CAD build for the part. Positions are in the model's coordinates, mm. Face numbers are marked on the shaded views. A direction names the side the tool comes from. Coordinates: 2 decimals unless noted, no trailing zeros. Write each loop counter-clockwise with the first axis right and the second up, starting at its lowest first coordinate (ties: lowest second). Pieces come first, ordered by that corner, then holes. Notation, with made-up numbers: M 0,31 L 38,31 A13 ccw 38,43 Z; hole C 18,60.25 d7. An arc over 180 degrees is marked long. Put each result on its own line as item: value. Start each with the question number.
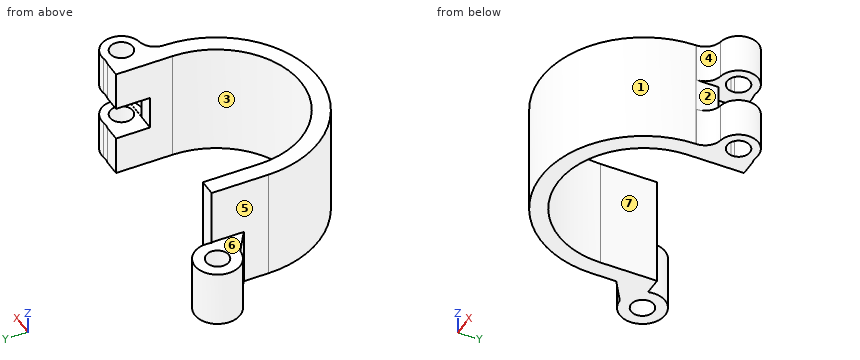
```python
from build123d import *

# Parameters (mm, degrees)
SKETCH1_R                           = 4
SKETCH1_R_2                         = 2
BOSS_EXTRUDE1_DEPTH                 = 10
BOSS_EXTRUDE2_DEPTH                 = 20
BOSS_EXTRUDE3_DEPTH                 = 10
SKETCH5_R                           = 3.5
SKETCH5_R_2                         = 2
BOSS_EXTRUDE4_DEPTH                 = 20
SKETCH4_W                           = 6
SKETCH4_H                           = 6.000142194
CUT_EXTRUDE1_DEPTH                  = 3
CUT_EXTRUDE1_DIRECTION_2_REACH      = 323.185
CUT_EXTRUDE1_DIRECTION_2_END_RADIUS = 3.5
FILLET2_R                           = 3
SKETCH6_W                           = 4.423537042
SKETCH6_H                           = 5.967206981
CUT_EXTRUDE2_DEPTH                  = 36.49639057
BODY_MOVE_COPY1_OUTLINE_R           = 2
BODY_MOVE_COPY1_DEPTH               = 10
BODY_MOVE_COPY1_START               = 2.967206981
BODY_MOVE_COPY1_2_DEPTH             = 0.032793019
BODY_MOVE_COPY1_START_2             = -10
BODY_MOVE_COPY1_3_OUTLINE_R         = 2
BODY_MOVE_COPY1_3_DEPTH             = 10
BODY_MOVE_COPY1_START_3             = -3
BODY_MOVE_COPY1_4_DEPTH             = 0.032793019


# Read off the part's stored shape, not the designer's step: Body-Move/Copy1
with BuildPart() as part:
    # Sketch1 → Boss-Extrude1 (new body)
    with BuildSketch(Plane.XY):
        with Locations(Location((-22, -289, 0), (0, 0, 270))):
            Circle(SKETCH1_R)
        with Locations(Location((-22, -289, 0), (0, 0, 270))):
            Circle(SKETCH1_R_2, mode=Mode.SUBTRACT)
    extrude(amount=BOSS_EXTRUDE1_DEPTH)



with BuildPart() as body_2:
    # Sketch2 → Boss-Extrude2 (new body)
    with BuildSketch(Plane.XY.offset(10)):
        with BuildLine():
            Line((-18, -300), (-18, -295.71047836))
            Line((-18, -295.71047836), (-18, -290))
            Line((-18, -290), (-15, -290))
            Line((-15, -290), (-15, -300))
            ThreePointArc((-15, -300), (0, -315), (15, -300))
            Line((15, -300), (15, -290))
            Line((15, -290), (18, -290))
            Line((18, -290), (18, -300))
            ThreePointArc((18, -300), (0, -318), (-18, -300))
        make_face()
    extrude(amount=-BOSS_EXTRUDE2_DEPTH)


with BuildPart() as part_1:
    add(part.part)

    add(body_2.part)  # Boss-Extrude3 merges body 2
    # Sketch3 → Boss-Extrude3 (add)
    with BuildSketch(Plane.XY.offset(10)):
        Polygon((-18, -290), (-18.290403154, -290), (-22, -293), (-18, -295.669919522), align=None)
    extrude(amount=-BOSS_EXTRUDE3_DEPTH)

    # Sketch5 → Boss-Extrude4 (add)
    with BuildSketch(Plane.XY.offset(10)):
        with Locations((19.974192434, -293.5)):
            Circle(SKETCH5_R)
        with Locations((19.974192434, -293.5)):
            Circle(SKETCH5_R_2, mode=Mode.SUBTRACT)
    extrude(amount=-BOSS_EXTRUDE4_DEPTH)

    # Sketch4 → Cut-Extrude1 (cut)
    with BuildSketch(Plane(origin=(18, 0, 0), x_dir=(0, 0, -1), z_dir=(1, 0, 0))):
        with Locations((0, -293.000071097)):
            Rectangle(SKETCH4_W, SKETCH4_H)
    extrude(amount=-CUT_EXTRUDE1_DEPTH, mode=Mode.SUBTRACT)

    # Cut-Extrude1 direction 2: up to this cylinder (the profile starts inside it)
    cut_extrude1_direction_2_end = Plane(origin=(19.974192434, -293.5, 0), z_dir=(0, 0, 1)) * Cylinder(CUT_EXTRUDE1_DIRECTION_2_END_RADIUS, 654.37, mode=Mode.PRIVATE)
    # Sketch4 → Cut-Extrude1 direction 2 (cut, up to the surface)
    with BuildSketch(Plane(origin=(18, 0, 0), x_dir=(0, 0, -1), z_dir=(1, 0, 0)), mode=Mode.PRIVATE) as cut_extrude1_direction_2_sk1:
        with Locations((0, -293.000071097)):
            Rectangle(SKETCH4_W, SKETCH4_H)
    cut_extrude1_direction_2_tool1 = extrude(cut_extrude1_direction_2_sk1.sketch, amount=CUT_EXTRUDE1_DIRECTION_2_REACH, mode=Mode.PRIVATE) & cut_extrude1_direction_2_end
    add(cut_extrude1_direction_2_tool1.solids().sort_by_distance((18, -293.000071, 0))[0], mode=Mode.SUBTRACT)

    # Fillet2
    # the kernel refuses this fillet: 3 mm, written as the material it adds along each edge
    with BuildSketch(Plane(origin=(18, -290.609919684, -10), x_dir=(1.5610699103436222e-12, 1.0, 0), z_dir=(0, 0, 1)), Plane(origin=(18, -290.609919684, 3), x_dir=(1.5610699103436222e-12, 1.0, 0), z_dir=(0, 0, 1))) as fillet2_piece_1:
        with BuildLine():
            CenterArc((3.502304969, -0.796308584), FILLET2_R, 164.60712684, 25.833288924)
            Line((0.551973299, -1.339947284), (0.492966665, -1.350820058))
            ThreePointArc((0.492966665, -1.350820058), (0.29061984, -0.663945695), (-0.049544234, -0.033843299))
            Line((-0.049544234, -0.033843299), (0, 0.06))
            ThreePointArc((0, 0.06), (0.304959842, 0.06), (0.552071978, 0.015926172))
            Line((0.552071978, 0.015926172), (0.609919684, 0))
        make_face()
    extrude(amount=7)
    with BuildSketch(Plane(origin=(18, -296.390080316, -10), x_dir=(0.975809068162025, -0.21862447825611958, 0), z_dir=(0, 0, 1))) as fillet2_piece_2:
        with BuildLine():
            CenterArc((3.698835937, -2.787234318), FILLET2_R, 111.708438384, 80.919816446)
            Line((0.771408732, -3.443107753), (0.712860188, -3.456225222))
            Line((0.712860188, -3.456225222), (-0.058548544, -0.013117469))
            Line((-0.058548544, -0.013117469), (0.022193016, 0.055744686))
            ThreePointArc((0.022193016, 0.055744686), (1.294592578, -0.188226629), (2.56699214, 0.055744686))
            Line((2.56699214, 0.055744686), (2.589185156, 0))
        make_face()
    extrude(amount=20)

    # Sketch6 → Cut-Extrude2 (cut, through all)
    with BuildSketch(Plane(origin=(0, -296.000142194, 0), x_dir=(1, 0, 0), z_dir=(0, 1, 0))):
        with Locations((20.211768521, 0.016396509)):
            Rectangle(SKETCH6_W, SKETCH6_H)
    extrude(amount=-CUT_EXTRUDE2_DEPTH, mode=Mode.SUBTRACT)

    # Body-Move/Copy1 outline → Body-Move/Copy1 (cut)
    with BuildSketch(Plane.XY):
        with BuildLine():
            Line((-18, -290), (-18.127016654, -290))
            ThreePointArc((-18.127016654, -290), (-24.449489743, -285.83772234), (-22, -293))
            Line((-22, -293), (-18, -295.669919522))
            Line((-18, -295.669919522), (-18, -290))
        make_face()
        with Locations((-22, -289)):
            Circle(BODY_MOVE_COPY1_OUTLINE_R, mode=Mode.SUBTRACT)
    extrude(amount=BODY_MOVE_COPY1_DEPTH, mode=Mode.SUBTRACT)

    # Body-Move_Copy1 2 outline → Body-Move_Copy1 2 (cut)
    with BuildSketch(Plane.XY.offset(BODY_MOVE_COPY1_START)):
        with BuildLine():
            ThreePointArc((20.526550354, -296.95613957), (21.549323306, -296.625533992), (22.423537042, -296.000142194))
            Line((22.423537042, -296.000142194), (18, -296.000142194))
            Line((18, -296.000142194), (18, -299.918544916))
            ThreePointArc((18, -299.918544916), (18.71741934, -297.971797492), (20.526550354, -296.95613957))
        make_face()
    extrude(amount=BODY_MOVE_COPY1_2_DEPTH, mode=Mode.SUBTRACT)

    # Body-Move_Copy1 3 outline → Body-Move_Copy1 3 (add)
    with BuildSketch(Plane.XY.offset(BODY_MOVE_COPY1_START_2)):
        with BuildLine():
            Line((-18, -290), (-18.127016654, -290))
            ThreePointArc((-18.127016654, -290), (-24.449489743, -285.83772234), (-22, -293))
            Line((-22, -293), (-18, -295.669919522))
            Line((-18, -295.669919522), (-18, -290))
        make_face()
        with Locations((-22, -289)):
            Circle(BODY_MOVE_COPY1_3_OUTLINE_R, mode=Mode.SUBTRACT)
    extrude(amount=BODY_MOVE_COPY1_3_DEPTH)

    # Body-Move_Copy1 4 outline → Body-Move_Copy1 4 (add)
    with BuildSketch(Plane.XY.offset(BODY_MOVE_COPY1_START_3)):
        with BuildLine():
            ThreePointArc((20.526550354, -296.95613957), (21.549323306, -296.625533992), (22.423537042, -296.000142194))
            Line((22.423537042, -296.000142194), (18, -296.000142194))
            Line((18, -296.000142194), (18, -299.918544916))
            ThreePointArc((18, -299.918544916), (18.71741934, -297.971797492), (20.526550354, -296.95613957))
        make_face()
    extrude(amount=BODY_MOVE_COPY1_4_DEPTH)


solid = part_1.part
```
(1) Slice it at C-C, the plane z = -8.25. Write the cut outline in (x, y), then the cut area to 3 significant figures.
(2) Drop flat-ended pins along their axis: pin 1 (0.9 mm diameter, centred on x = 16.5, z = 6, fed in from +Y); pin 2 (10 mm diameter, centred on y = -306.5, z = -5, fed in from +X); pin 3 (3 mm diameter, centred on x = -22, y = -289, fed in from +Z); pin 4 (1.2 mm diameter, centred on y = -298.5, z = 1.5, fed in from +X). Give the stop position or say it passes through.
(3) Which spindle directions (+Z, -Z, +X, -X, +Y, -Y) get a long thin tool onto all of the face, cutting with end or side? Do the marked faces 4, 5, 6 and 7. Say none if no direction does.
(4) Drill centre lines: line 1 (X direction, y = -293.5, z = 6.75); line 2 (X direction, y = -293.5, z = -6); line 3 (Y direction, x = -22, z = -4.25). Where is each one in solid material? Low to high. Write a range as [from, to].
(5) Two-plate mould, pull along X, no slides. Class the marked faces 1, 2 and 3: +X half, -X half, draft (parallel to the pull), parting line (faces both ways), or undercut.
(6) Slice it at A-A, the plane y = -289. Write the cut outline in (x, z).
(7) Slice it at D-D, the plane x = 0. Write the cut outline in (y, z), then the cut area to 3 significant figures.
(8) Slice it at B-B, the plane z = -0.75. Write the cut outline in (x, y).
Result set:
1. outline: M -22,-293 L -18,-295.67 L -18,-300 A18 ccw 18,-300 L 18,-299.92 A3 cw 20.53,-296.96 A3.5 ccw long 19.34,-290.06 A3 cw 18,-290 L 15,-290 L 15,-300 A15 cw -15,-300 L -15,-290 L -18.13,-290 A4 ccw long Z; hole C -22,-289 d4; hole M 18,-293.82 A2 ccw long 18,-293.18 Z
1. area: 284 mm^2
2. pin 1: stops at y = -290
2. pin 2: stops at x = 17.94
2. pin 3: passes through
2. pin 4: stops at x = 18
3. face 4: +Z, -Z, +X, -Y
3. face 5: +Z, -X, -Y
3. face 6: +Z, -X, +Y, -Y
3. face 7: +Z, -Z, +Y
4. line 1: x = [-18, -15], [15, 18], [21.97, 23.47]
4. line 2: x = [-21.25, -15], [15, 18], [21.97, 23.47]
4. line 3: y = [-293, -291], [-287, -285]
5. face 1: parting line
5. face 2: +X half
5. face 3: undercut
6. outline: M -26,-10 L -24,-10 L -24,0 L -26,0 Z; M -20,-10 L -18,-10 L -18,0 L -20,0 Z
7. outline: M -318,-10 L -315,-10 L -315,10 L -318,10 Z
7. area: 60.0 mm^2
8. outline: M -22,-293 L -18,-295.67 L -18,-300 A18 ccw 18,-300 L 18,-296 L 15,-296 L 15,-300 A15 cw -15,-300 L -15,-290 L -18.13,-290 A4 ccw long Z; hole C -22,-289 d4
